from build123d import *

# Parameters (mm, degrees)
BASE_FLANGE_DEPTH         = 31.75
MITER_FLANGE2_DEPTH       = 88.9
MITER_FLANGE2_2_DEPTH     = 3.175
MITER_START               = 3.175
MITER_FLANGE2_3_DEPTH     = 85.725
MITER_START_2             = -19.05
MITER_FLANGE2_4_OUTLINE_W = 19.05
MITER_FLANGE2_4_OUTLINE_H = 1.5875
MITER_FLANGE2_4_DEPTH     = 17.4625
MITER_FLANGE2_5_DEPTH     = 19.05
MITER_FLANGE2_6_DEPTH     = 19.05
CUT_EXTRUDE1_REACH        = 105.029
SKETCH4_R                 = 2.54
CUT_EXTRUDE2_REACH        = 105.029
SKETCH5_R                 = 2.54
CUT_EXTRUDE4_REACH        = 107.049
SKETCH7_R                 = 2.54


with BuildPart() as part:
    # Base-Flange: sheet metal written as solids
    # Sketch1 → Base-Flange (new body)
    with BuildSketch(Plane.XY):
        with BuildLine():
            Line((0, 0), (19.05, 0))
            ThreePointArc((19.05, 0), (21.29506403, 0.92993597), (22.225, 3.175))
            Line((22.225, 3.175), (22.225, 88.9))
            Line((22.225, 88.9), (20.6375, 88.9))
            Line((20.6375, 88.9), (20.6375, 3.175))
            ThreePointArc((20.6375, 3.175), (20.172532015, 2.052467985), (19.05, 1.5875))
            Line((19.05, 1.5875), (0, 1.5875))
            Line((0, 1.5875), (0, 0))
        make_face()
    extrude(amount=BASE_FLANGE_DEPTH)

    # Miter Flange2: read off the stored shape, not the designer's step
    # Miter Flange2 outline → Miter Flange2 (cut)
    with BuildSketch(Plane(origin=(0, 0, 0), x_dir=(1, 0, 0), z_dir=(0, 1, 0))):
        with BuildLine():
            Line((22.225, 0), (19.05, 0))
            Line((19.05, 0), (19.05, -3.175))
            Line((19.05, -3.175), (20.6375, -3.175))
            ThreePointArc((20.6375, -3.175), (21.062869343, -1.5875), (22.225, -0.425369343))
            Line((22.225, -0.425369343), (22.225, 0))
        make_face()
    extrude(amount=MITER_FLANGE2_DEPTH, mode=Mode.SUBTRACT)

    # Miter Flange2 2 outline → Miter Flange2 2 (cut)
    with BuildSketch(Plane(origin=(0, 0, 0), x_dir=(1, 0, 0), z_dir=(0, 1, 0))):
        with BuildLine():
            Line((20.6375, -3.175), (22.225, -3.175))
            Line((22.225, -3.175), (22.225, -0.425369343))
            ThreePointArc((22.225, -0.425369343), (21.062869343, -1.5875), (20.6375, -3.175))
        make_face()
    extrude(amount=MITER_FLANGE2_2_DEPTH, mode=Mode.SUBTRACT)

    # Miter Flange2 3 outline → Miter Flange2 3 (add)
    with BuildSketch(Plane(origin=(0, 0, 0), x_dir=(1, 0, 0), z_dir=(0, 1, 0)).offset(MITER_START)):
        with BuildLine():
            Line((22.225, -0.425369343), (22.225, -3.175))
            ThreePointArc((22.225, -3.175), (22.689967985, -2.052467985), (23.8125, -1.5875))
            Line((23.8125, -1.5875), (41.275, -1.5875))
            Line((41.275, -1.5875), (41.275, 0))
            Line((41.275, 0), (23.8125, 0))
            ThreePointArc((23.8125, 0), (22.990749532, -0.108185502), (22.225, -0.425369343))
        make_face()
    extrude(amount=MITER_FLANGE2_3_DEPTH)

    # Miter Flange2 5 outline → Miter Flange2 5 (cut)
    with BuildSketch(Plane.YZ):
        with BuildLine():
            ThreePointArc((1.5875, 3.175), (1.162130657, 1.5875), (0, 0.425369343))
            Line((0, 0.425369343), (0, 0))
            Line((0, 0), (1.5875, 0))
            Line((1.5875, 0), (1.5875, 3.175))
        make_face()
    extrude(amount=MITER_FLANGE2_5_DEPTH, mode=Mode.SUBTRACT)



with BuildPart() as body_2:
    # Miter Flange2 4 outline → Miter Flange2 4 (new body)
    with BuildSketch(Plane(origin=(0, 0, 0), x_dir=(1, 0, 0), z_dir=(0, 1, 0)).offset(MITER_START_2)):
        with Locations((9.525, -0.79375)):
            Rectangle(MITER_FLANGE2_4_OUTLINE_W, MITER_FLANGE2_4_OUTLINE_H)
    extrude(amount=MITER_FLANGE2_4_DEPTH)


with BuildPart() as part_1:
    add(part.part)

    add(body_2.part)  # Miter Flange2 6 merges body 2
    # Miter Flange2 6 outline → Miter Flange2 6 (add)
    with BuildSketch(Plane.YZ):
        with BuildLine():
            Line((0, 0.425369343), (0, 3.175))
            ThreePointArc((0, 3.175), (-0.464967985, 2.052467985), (-1.5875, 1.5875))
            Line((-1.5875, 1.5875), (-1.5875, 0))
            ThreePointArc((-1.5875, 0), (-0.765749532, 0.108185502), (0, 0.425369343))
        make_face()
    extrude(amount=MITER_FLANGE2_6_DEPTH)

    # Sketch4 → Cut-Extrude1 (cut, up to next)
    with BuildSketch(Plane(origin=(0, 0, 0), x_dir=(-1, 0, 0), z_dir=(0, 0, -1)), mode=Mode.PRIVATE) as cut_extrude1_sk1:
        with Locations((-34.925, 76.2)):
            Circle(SKETCH4_R)
    cut_extrude1_tool1 = extrude(cut_extrude1_sk1.sketch, amount=-CUT_EXTRUDE1_REACH, mode=Mode.PRIVATE) & part_1.part
    # Sketch4 → Cut-Extrude1 (cut, up to next)
    with BuildSketch(Plane(origin=(0, 0, 0), x_dir=(-1, 0, 0), z_dir=(0, 0, -1)), mode=Mode.PRIVATE) as cut_extrude1_sk2:
        with Locations((-34.925, 46.0375)):
            Circle(SKETCH4_R)
    cut_extrude1_tool2 = extrude(cut_extrude1_sk2.sketch, amount=-CUT_EXTRUDE1_REACH, mode=Mode.PRIVATE) & part_1.part
    # Sketch4 → Cut-Extrude1 (cut, up to next)
    with BuildSketch(Plane(origin=(0, 0, 0), x_dir=(-1, 0, 0), z_dir=(0, 0, -1)), mode=Mode.PRIVATE) as cut_extrude1_sk3:
        with Locations((-34.925, 15.875)):
            Circle(SKETCH4_R)
    cut_extrude1_tool3 = extrude(cut_extrude1_sk3.sketch, amount=-CUT_EXTRUDE1_REACH, mode=Mode.PRIVATE) & part_1.part
    add(cut_extrude1_tool1.solids().sort_by_distance((34.925, 76.2, 0))[0], mode=Mode.SUBTRACT)
    add(cut_extrude1_tool2.solids().sort_by_distance((34.925, 46.0375, 0))[0], mode=Mode.SUBTRACT)
    add(cut_extrude1_tool3.solids().sort_by_distance((34.925, 15.875, 0))[0], mode=Mode.SUBTRACT)

    # Sketch5 → Cut-Extrude2 (cut, up to next)
    with BuildSketch(Plane(origin=(0, 0, 0), x_dir=(-1, 0, 0), z_dir=(0, 0, -1)), mode=Mode.PRIVATE) as cut_extrude2_sk1:
        with Locations((-12.7, -12.7)):
            Circle(SKETCH5_R)
    cut_extrude2_tool1 = extrude(cut_extrude2_sk1.sketch, amount=-CUT_EXTRUDE2_REACH, mode=Mode.PRIVATE) & part_1.part
    add(cut_extrude2_tool1.solids().sort_by_distance((12.7, -12.7, 0))[0], mode=Mode.SUBTRACT)

    # Sketch7 → Cut-Extrude4 (cut, up to next)
    with BuildSketch(Plane(origin=(22.225, -0.213353633, 50.991788494), x_dir=(0, 0, -1), z_dir=(1, 0, 0)), mode=Mode.PRIVATE) as cut_extrude4_sk1:
        with Locations(Location((25.591788494, 76.413353633, 0), (0, 0, 90))):
            Circle(SKETCH7_R)
    cut_extrude4_tool1 = extrude(cut_extrude4_sk1.sketch, amount=-CUT_EXTRUDE4_REACH, mode=Mode.PRIVATE) & part_1.part
    # Sketch7 → Cut-Extrude4 (cut, up to next)
    with BuildSketch(Plane(origin=(22.225, -0.213353633, 50.991788494), x_dir=(0, 0, -1), z_dir=(1, 0, 0)), mode=Mode.PRIVATE) as cut_extrude4_sk2:
        with Locations(Location((25.591788494, 46.250853633, 0), (0, 0, 90))):
            Circle(SKETCH7_R)
    cut_extrude4_tool2 = extrude(cut_extrude4_sk2.sketch, amount=-CUT_EXTRUDE4_REACH, mode=Mode.PRIVATE) & part_1.part
    # Sketch7 → Cut-Extrude4 (cut, up to next)
    with BuildSketch(Plane(origin=(22.225, -0.213353633, 50.991788494), x_dir=(0, 0, -1), z_dir=(1, 0, 0)), mode=Mode.PRIVATE) as cut_extrude4_sk3:
        with Locations(Location((25.591788494, 16.088353633, 0), (0, 0, 90))):
            Circle(SKETCH7_R)
    cut_extrude4_tool3 = extrude(cut_extrude4_sk3.sketch, amount=-CUT_EXTRUDE4_REACH, mode=Mode.PRIVATE) & part_1.part
    add(cut_extrude4_tool1.solids().sort_by_distance((22.225, 76.2, 25.4))[0], mode=Mode.SUBTRACT)
    add(cut_extrude4_tool2.solids().sort_by_distance((22.225, 46.0375, 25.4))[0], mode=Mode.SUBTRACT)
    add(cut_extrude4_tool3.solids().sort_by_distance((22.225, 15.875, 25.4))[0], mode=Mode.SUBTRACT)

    # SHM-Mirror1: part across plane


with BuildPart() as part_2:
    add(part_1.part)
    add(part_1.part.mirror(Plane(origin=(0, 0, 31.75), x_dir=(0, 0, 1), z_dir=(-1, 0, 0))))


solid = part_2.part
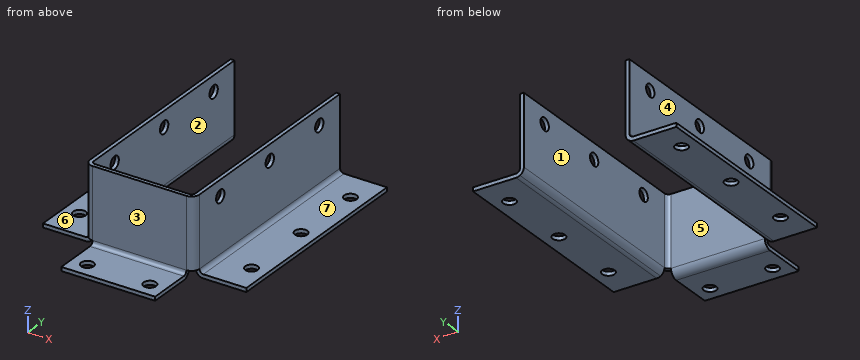
Verification items for the finished model (mm, model axes). Face numbers are marked on the shaded views. A direction names the side the tool comes from. Coordinates: 2 decimals unless noted, no trailing zeros. Write each loop counter-clockwise with the first axis right and the second up, starting at its lowest first coordinate (ties: lowest second). Pieces come first, ordered by that corner, then holes. Notation, with made-up numbers: (32.25, -34.75) -> (72.25, -34.75) arc R14 ccw to (72.25, -28.75) -> close; hole circle Ø7 at (72, -12). An arc over 180 degrees is marked (long way). One line per item, written item: value. Start each with the question number.
Q1. Thickness scan on L1, parallel to X at y = 18.5, z = 12 (1 decimal); L2, parallel to Z at x = -28, y = 14. Record the ranges inside material, lowest first. Write a range as from..to.
Q2. Cross-section at C-C on y = 76.2. State how many separate pieces and enclosed holes the cut face has, and give its area (3 significant figures).
Q3. Mould release check, pull along X, two halves, no side actions. Record for the marked faces 1, 2, 3 and 4: pulls with the +X half, pulls with the -X half, needs draft (parallel to the pull), parting line crosses it, or undercut.
Q4. Access from +Z, -Z, +X, -X, +Y, -Y to the whole of each face (thin tool, end or side, straight path). Record for the marked faces 5, 6 and 7.
Q5. Cross-section at A-A on y = -12.7. Enter the section's corners in (x, z), and give its area (3 significant figures).
Q6. Go/stop test with flat-tipped pins: P1, Ø6.5, axis at x = 34.925, y = 76.2, coming from the +Z side; P2, Ø4.5, axis at x = -34.92, y = 46.04, coming from the -Z side; P3, Ø4, axis at y = 62.5, z = 21, coming from the -X side (3 decimals); P4, Ø3.5, axis at x = 29.5, z = 2, coming from the -Y side (3 decimals). Record where each tip stops, or that it passes through.
Checked values:
1. L1: x = -22.2..-20.6, 20.6..22.2
1. L2: z = 0..1.59
2. separate pieces: 6
2. enclosed holes: 0
2. area: 126 mm²
3. face 1: undercut
3. face 2: undercut
3. face 3: needs draft
3. face 4: pulls with the -X half
4. face 5: +Z, -Z, +Y
4. face 6: +Z, -X, +Y, -Y
4. face 7: +Z, +X, +Y, -Y
5. outline: (-19.05, 0) -> (-15.24, 0) -> (-15.24, 1.59) -> (-19.05, 1.59) -> close; (-10.16, 0) -> (10.16, 0) -> (10.16, 1.59) -> (-10.16, 1.59) -> close; (15.24, 0) -> (19.05, 0) -> (19.05, 1.59) -> (15.24, 1.59) -> close
5. area: 44.4 mm²
6. P1: stops at z = 1.59
6. P2: passes through
6. P3: stops at x = -22.225
6. P4: stops at y = 3.175
